Autodesk Inventor part; units mm, degrees
ref_plane "YZ Plane" through (0, 0, 0) normal (1, 0, 0) x (0, 1, 0)
ref_plane "XZ Plane" through (0, 0, 0) normal (0, 1, 0) x (-1, 0, 0)
ref_plane "XY Plane" through (0, 0, 0) normal (0, 0, 1) x (1, 0, 0)
sketch "Sketch1" plane through (0, 0, 0) normal (0, 0, 1) x (1, 0, 0)
  line L0 (0, 0) -> (24, 0)
  line L1 (24, 0) -> (24, -60)
  line L2 (24, -60) -> (0, -60)
  line L3 (0, -60) -> (0, 0)
  dimension "d0" = 24
  dimension "d1" = 60
extrude "Extrusion1" add sketch "Sketch1" along normal blind 2
sketch "Sketch2" plane through (0, 0, 2) normal (0, 0, 1) x (1, 0, 0)
  line L0 (0, -60) -> (24, -60)
  line L1 (0, 0) -> (2, 0)
  line L2 (2, 0) -> (2, -60)
  line L3 (2, -60) -> (0, -60)
  line L4 (0, -60) -> (0, 0)
  line L5 (24, -60) -> (24, 0)
  line L6 (24, 0) -> (22, 0)
  line L7 (22, 0) -> (22, -60)
  line L8 (22, -60) -> (24, -60)
  line L9 (24, -60) -> (24, 0)
  dimension "d4" = 2
  dimension "d5" = 2
extrude "Extrusion2" add sketch "Sketch2" along normal blind 15
sketch "Sketch3" plane through (24, -60, 0) normal (1, 0, 0) x (0, 0, -1)
  circle A0 centre (-8.5, 57) radius 1
  circle A1 centre (-8.5, 29.5) radius 1
  line L0 (-17, 0) -> (-17, 60)
  line L1 (0, 60) -> (-17, 60)
  dimension "d8" = 2
  dimension "d9" = 2
  dimension "d10" = 8.5
  dimension "d11" = 8.5
  dimension "d12" = 27.5
  dimension "d13" = 3
extrude "Extrusion3" cut sketch "Sketch3" against normal up to surface (2 mm away)
sketch "Sketch4" plane through (24, -60, 0) normal (1, 0, 0) x (0, 0, -1)
  line L0 (-17, 60) -> (-17, 0)
  line L1 (-17, 55) -> (-2, 55)
  line L2 (-2, 55) -> (-2, 31.5)
  line L3 (-2, 31.5) -> (-17, 31.5)
  line L4 (-17, 31.5) -> (-17, 55)
  circle A0 centre (-8.5, 57) radius 1
  circle A1 centre (-8.5, 29.5) radius 1
  point P0 (-17, 31.5)
  dimension "d23" = 15
  dimension "d24" = 23.5
  dimension "d25" = 2
  dimension "d26" = 2
extrude "Extrusion4" cut sketch "Sketch4" against normal up to surface (2 mm away) contours L1 L2 L3 L0
sketch "Sketch5" plane through (0, -60, 0) normal (-1, 0, 0) x (0, 0, 1)
  circle A0 centre (8.5, 48.4) radius 2.5
  circle A1 centre (8.5, 57) radius 1
  point P0 (0, 60)
  dimension "d29" = 5
  dimension "d32" = 8.6
  dimension "d33" = 0
extrude "Extrusion5" add sketch "Sketch5" along normal blind 5 contours A0
sketch "Sketch6" plane through (2, -60, 2) normal (1, 0, 0) x (0, 0, -1)
  line L0 (2, 60) -> (-15, 60)
  line L1 (2, 0) -> (-15, 0)
  line L2 (-15, 60) -> (-13, 60)
  line L3 (-13, 60) -> (-13, 0)
  line L4 (-13, 0) -> (-15, 0)
  line L5 (-15, 0) -> (-15, 60)
  dimension "d34" = 2
extrude "Extrusion6" add sketch "Sketch6" along normal up to surface (22 mm away)
sketch "Sketch7" plane through (0, 0, 0) normal (0, 0, -1) x (-1, 0, 0)
  line L0 (-24, -5) -> (-22, -5)
  line L1 (-24, -5) -> (-22, -5)
  line L2 (-22, -5) -> (-22, -28.5)
  line L3 (-22, -28.5) -> (-24, -28.5)
  line L4 (-24, -28.5) -> (-24, -5)
  line L5 (-2, -60) -> (-22, -60)
  line L6 (-22, 0) -> (-2, 0)
  line L7 (-2, 0) -> (-2, -60)
  line L8 (-2, -60) -> (-22, -60)
  line L9 (-22, -60) -> (-22, 0)
  point P0 (0, -60)
  point P1 (-22, -5)
  point P2 (-22, -28.5)
  point P3 (-22, -60)
extrude "Extrusion7" cut sketch "Sketch7" against normal up to surface (2 mm away)
sketch "Sketch8" plane through (22, -60, 0) normal (0, -1, 0) x (1, 0, 0)
  line L0 (-20, 15) -> (0, 15)
  line L1 (0, 15) -> (0, 0)
  line L2 (0, 0) -> (-20, 0)
  line L3 (-20, 0) -> (-20, 15)
  point P0 (-22, 0)
extrude "Extrusion8" add sketch "Sketch8" against normal blind 10.5
sketch "Sketch9" plane through (0, 0, 0) normal (0, 1, 0) x (1, 0, 0)
  line L0 (24, -17) -> (0, -17)
  line L1 (0, -17) -> (0, 0)
  line L2 (0, 0) -> (24, 0)
  line L3 (24, 0) -> (24, -17)
extrude "Extrusion9" add sketch "Sketch9" along normal blind 2
fillet "Fillet1" radius 8.5 4 edges at (12, -60, 17) (0, -60, 8.5) (12, -60, 0) (24, -60, 8.5)
sketch "Sketch10" plane through (0, 2, 0) normal (0, 1, 0) x (1, 0, 0)
  circle A0 centre (12, -8.5) radius 6
  line L0 (0, 0) -> (0, -17)
  line L1 (0, -17) -> (24, -17)
  dimension "d45" = 12
  dimension "d46" = 12
  dimension "d47" = 8.5
extrude "Extrusion10" cut sketch "Sketch10" against normal up to surface (2 mm away)
properties part number "juncao4"
Part model, mm, in its own coordinate system. A direction names the side the tool comes from. Give positions to 0.01 mm unless a question says otherwise; leave off trailing zeros. Order: outer loops, then holes, each group sorted by start corner. A loop starts at its lowest first (then second) coordinate and runs counter-clockwise, first axis right, second up. Notation, with made-up numbers: (68.5, 71) - (80.5, 71) arc R14 ccw to (80.5, 81) - close; hole circle Ø2 at (67.25, 50.5). An arc over 180 degrees is marked (long way). Use one line per item in the form item = value.
Item 1: Pin check, flat tips, straight feed: pin 1 Ø8 at (y, z) = (-37, 6.5) entering from -X; pin 2 Ø1 at (x, z) = (13.5, 10.5) entering from +Y; pin 3 Ø1.5 at (x, y) = (17.5, -44.5) entering from -Z. Stop position of each tip, or through.
Solution:
pin_1 = 0
pin_2 = -49.5
pin_3 = 15
Item 2: Probe probe 1 along Y at (x, z) = (22.55, 8.5); probe 2 along Y at (x, z) = (22.5, 8.5); probe 3 along X at (y, z) = (-3.5, 4.75). List the from-to ranges inside material, lowest first. Write a range as from..to.
Solution:
probe_1 = -56.25..-31.5, -29.5..-28.5, -5..-4, -2..2
probe_2 = -56.32..-31.5, -29.5..-28.5, -5..-4, -2..2
probe_3 = 0..2, 22..24
Item 3: Which spindle directions (+Z, -Z, +X, -X, +Y, -Y) get a long thin tool onto all of the face, cutting with end or side? Do faces 1 (the face through (24, -31, 10)), 2 (the face through (22, -2, 7)), 3 (the face through (22.41, -56.45, 8.62)), 4 (the face through (-2.465, -12.351, 10.885)), 5 (the face through (23, -3.6, 9.3)). Say none if no direction does.
Solution:
face_1 = +Z, -Z, +X, +Y, -Y
face_2 = -Z
face_3 = +Z, -Z, +X, -Y
face_4 = -X
face_5 = +X
Item 4: Slice it at B-B on z = 12.25. Give the cut face in (x, y), and give its area (3 significant figures).
Solution:
outline = (0, -51.5) arc R8.5 ccw to (4.75, -59.13) - (19.25, -59.13) arc R8.5 ccw to (24, -51.5) - (24, -28.5) - (22, -28.5) - (22, -49.5) - (2, -49.5) - (2, 0) - (7.32, 0) - (7.32, 2) - (0, 2) - close; (16.68, 0) - (22, 0) - (22, -5) - (24, -5) - (24, 2) - (16.68, 2) - close
area = 391 mm2
Item 5: Two-plate mould, pull along X, no slides. Class faces 6 (the face through (2, -24, 7)), 7 (the face through (1.484, -56.299, 8.619)), 8 (the face through (12, 0, 2)), 9 (the face through (1, -25, 0)): released by +X, released by -X, zero draft, split by the parting line, or undercut.
Solution:
face_6 = undercut
face_7 = released by -X
face_8 = undercut
face_9 = zero draft
Item 6: Slice it at A-A on y = -30.5. Give the cut face in (x, z), and give its area (3 significant figures).
Solution:
outline = (0, 0) - (2, 0) - (2, 15) - (22, 15) - (22, 9.5) - (24, 9.5) - (24, 17) - (0, 17) - close; (22, 0) - (24, 0) - (24, 7.5) - (22, 7.5) - close
area = 104 mm2
Item 7: Slice it at C-C on x = 7.75. Give the cut face in (y, z), and give its area (3 significant figures).
Solution:
outline = (-59.97, 7.75) arc R8.5 ccw to (-51.5, 0) - (-49.5, 0) - (-49.5, 15) - (0, 15) - (0, 12.74) - (2, 12.74) - (2, 17) - (-51.5, 17) arc R8.5 ccw to (-59.97, 9.25) - close; (0, 0) - (2, 0) - (2, 4.26) - (0, 4.26) - close
area = 264 mm2
Item 8: Slice it at D-D on y = -11.6. Give the cut face in (x, z), and give its area (3 significant figures).
Solution:
outline = (-5, 6) - (0, 6) - (0, 0) - (2, 0) - (2, 15) - (24, 15) - (24, 17) - (0, 17) - (0, 11) - (-5, 11) - close
area = 103 mm2
